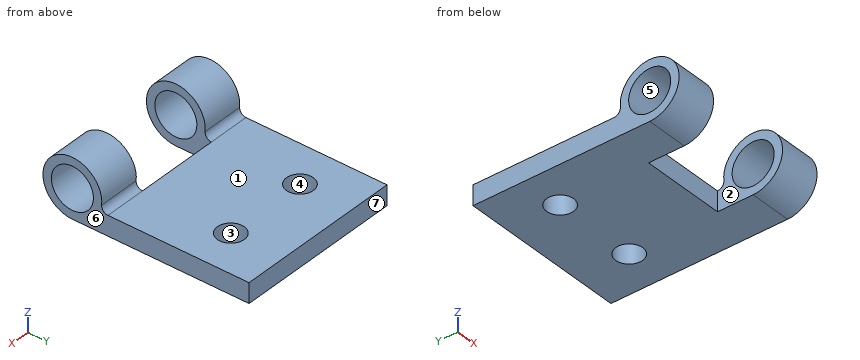
```python
from build123d import *

# Parameters (mm, degrees)
SKETCH2_R               = 1.5875
BOSS_EXTRUDE1_DEPTH     = 12.7
SKETCH3_R               = 1.016
CUT_EXTRUDE1_DEPTH      = 12.7
CUT_EXTRUDE3_DEPTH      = 5.08
CUT_EXTRUDE3_DEPTH_BACK = 50.8
SKETCH4_W               = 6.35
SKETCH4_H               = 4.911764537
SCALE1_SCALE            = 3


with BuildPart() as part:
    # Sketch2 → Boss-Extrude1 (new body)
    with BuildSketch(Plane(origin=(0, 0, 0), x_dir=(0, 0, -1), z_dir=(1, 0, 0))):
        with BuildLine():
            Line((0.7234417, 2.689264537), (0.7234417, 13.340138709))
            Line((0.7234417, 13.340138709), (2.2225, 13.340138709))
            Line((2.2225, 13.340138709), (2.2225, 0))
            ThreePointArc((2.2225, 0), (-1.641425032, -1.498409194), (0.202045455, 2.213297062))
            ThreePointArc((0.202045455, 2.213297062), (0.567726646, 2.33627761), (0.7234417, 2.689264537))
        make_face()
        Circle(SKETCH2_R, mode=Mode.SUBTRACT)
    extrude(amount=BOSS_EXTRUDE1_DEPTH)

    # Sketch3 → Cut-Extrude1 (cut)
    with BuildSketch(Plane.XY.offset(-0.7234417)):
        with Locations((3.168860155, 9.364146191)):
            Circle(SKETCH3_R)
        with Locations((9.531139845, 9.364146191)):
            Circle(SKETCH3_R)
    extrude(amount=-CUT_EXTRUDE1_DEPTH, mode=Mode.SUBTRACT)

    # Sketch4 → Cut-Extrude3 (cut, two sides: drawn at the far end of the back side and taken through both)
    with BuildSketch(Plane.XY.offset(-0.7234417).offset(-CUT_EXTRUDE3_DEPTH_BACK)):
        with Locations((6.35, 0.233382268)):
            Rectangle(SKETCH4_W, SKETCH4_H)
    extrude(amount=CUT_EXTRUDE3_DEPTH + CUT_EXTRUDE3_DEPTH_BACK, mode=Mode.SUBTRACT)


with BuildPart() as part_1:
    # Scale1: scaled about (6.35, 6.161123686, -1.197561497)
    add(part.part.scale(SCALE1_SCALE).moved(Location((-12.7, -12.322247372, 2.395122994))))


solid = part_1.part
```
Input: part model. Units: mm. Frame: model coordinates. Face numbers are marked on the shaded views. A direction names the side the tool comes from. Coordinates: 2 decimals unless noted, no trailing zeros. Write each loop counter-clockwise with the first axis right and the second up, starting at its lowest first coordinate (ties: lowest second). Pieces come first, ordered by that corner, then holes. Notation, with made-up numbers: (-15, 85.25) - (44, 85.25) arc R15 cw to (44, 98.25) - close; hole circle Ø3 at (26, 61). An arc over 180 degrees is marked (long way). Put each result on its own line as item: value. Start each with the question number.
1) Ray query, L1, parallel to Y at x = -6, z = 2.5; L2, parallel to X at y = -8, z = -2.25 (3 decimals); L3, parallel to Z at x = -10, y = 19. Return the intervals inside material, ascending.
2) Cut plane B-B (y = 17). Return the cut outline in (x, z).
3) Contact query for flat-ended pins moving along their axis: pin 1 (1.5 mm diameter, centred on x = -1, y = -5.5, fed in from -Z); pin 2 (10 mm diameter, centred on x = 15.89, y = 15.77, fed in from +Z); pin 3 (7 mm diameter, centred on x = -3.19, y = 15.77, fed in from -Z); pin 4 (5 mm diameter, centred on x = 6.5, z = -2, fed in from -Y). Output: stop coordinate, or through.
4) Cut plane A-A (z = 3). Return the cut outline in (x, y) (3 decimals), plus the area to 3 significant figures.
5) Cut plane C-C (x = 16.5). Return the cut outline in (y, z) (1 decimal).
6) Cut plane D-D (z = -0.5). Return the cut outline in (x, y) (3 decimals).
7) Reachability of the marked faces 1, 2 and 3 from +Z, -Z, +X, -X, +Y, -Y: full face, straight path, thin tool, end or side. Return the list, or none.
8) Mould query, pull axis Y, two halves, no side actions, for the marked faces 4, 5, 6 and 7. Classes: pulls with the +Y half, pulls with the -Y half, needs draft (parallel to the pull), parting line crosses it, or undercut.
Resolved:
1. L1: y = -18.99 to -17.08, -7.56 to -5.66
1. L2: x = -12.7 to -3.175, 15.875 to 25.4
1. L3: z = -4.27 to 0.22
2. outline: (-12.7, -4.27) - (-5.98, -4.27) - (-5.98, 0.22) - (-12.7, 0.22) - close; (-0.4, -4.27) - (13.1, -4.27) - (13.1, 0.22) - (-0.4, 0.22) - close; (18.68, -4.27) - (25.4, -4.27) - (25.4, 0.22) - (18.68, 0.22) - close
3. pin 1: passes through
3. pin 2: stops at z = 0.22
3. pin 3: stops at z = -4.27
3. pin 4: stops at y = -4.25
4. outline: (-12.7, -18.962) - (-3.175, -18.962) - (-3.175, -17.046) - (-12.7, -17.046) - close; (-12.7, -7.598) - (-3.175, -7.598) - (-3.175, -5.682) - (-12.7, -5.682) - close; (15.875, -18.962) - (25.4, -18.962) - (25.4, -17.046) - (15.875, -17.046) - close; (15.875, -7.598) - (25.4, -7.598) - (25.4, -5.682) - (15.875, -5.682) - close
4. area: 73.0 mm2
5. outline: (-12.3, -4.3) - (12.8, -4.3) - (12.8, 0.2) - (-4.3, 0.2) arc R1.4 cw to (-5.7, 1.8) arc R6.7 ccw (long way) to start; (18.8, -4.3) - (27.7, -4.3) - (27.7, 0.2) - (18.8, 0.2) - close; hole circle Ø9.5 at (-12.3, 2.4)
6. outline: (-12.7, -18.328) - (-3.175, -18.328) - (-3.175, -16.104) - (-12.7, -16.104) - close; (-12.7, -8.541) - (-3.175, -8.541) - (-3.175, -4.254) - (15.875, -4.254) - (15.875, -8.541) - (25.4, -8.541) - (25.4, 27.698) - (-12.7, 27.698) - close; (15.875, -18.328) - (25.4, -18.328) - (25.4, -16.104) - (15.875, -16.104) - close; hole circle Ø6.096 at (-3.193, 15.77); hole circle Ø6.096 at (15.893, 15.77)
7. face 1: +Z, +X, -X, +Y
7. face 2: +Z, -Z, -Y
7. face 3: +Z, -Z
8. face 4: undercut
8. face 5: undercut
8. face 6: needs draft
8. face 7: pulls with the +Y half
